Geometry: final body of the model. Coordinates: model frame, mm. Face numbers are marked on the shaded views. Round coordinates to 2 decimals unless told otherwise and drop trailing zeros. Loops run counter-clockwise (first coordinate to the right, second up) from the corner with the lowest first, then second, coordinate; pieces in that order, holes last. Notation, with made-up numbers: (-36.75, 62.5) -> (10.25, 62.5) arc R16 ccw to (10.25, 67.5) -> close; hole circle Ø9 at (48, -36.5). An arc over 180 degrees is marked (long way). Answer in a Markdown table with one row per item.
```python
from build123d import *

# Parameters (mm, degrees)
SKETCH2_R             = 7.9375
SKETCH2_R_2           = 3.8862
BOSS_EXTRUDE1_DEPTH   = 6.35
SKETCH2_R_3           = 1.70815
BOSS_EXTRUDE1_2_DEPTH = 6.35
BOSS_EXTRUDE3_START   = -2.54
SKETCH2_6_R           = 7.9375
SKETCH2_6_R_2         = 1.70815
BOSS_EXTRUDE3_DEPTH   = 2.54
CHAMFER2_SIZE         = 1.27
CHAMFER2_SIZE2        = 1.513527063
CHAMFER3_SIZE         = 0.635


with BuildPart() as part:
    # Sketch2 → Boss-Extrude1 (new body)
    with BuildSketch(Plane(origin=(0, 0, 0), x_dir=(0, 1, 0), z_dir=(0, 0, 1))):
        with Locations(Location((0, 0, 0), (0, 0, 270))):
            Circle(SKETCH2_R)
        with Locations(Location((0, 0, 0), (0, 0, 270))):
            Circle(SKETCH2_R_2, mode=Mode.SUBTRACT)
    extrude(amount=BOSS_EXTRUDE1_DEPTH)

    # Sketch2<6> → Boss-Extrude3 (add)
    with BuildSketch(Plane(origin=(0, 0, 0), x_dir=(0, 1, 0), z_dir=(0, 0, 1)).offset(BOSS_EXTRUDE3_START)):
        with Locations(Location((0, 0, 0), (0, 0, 270))):
            Circle(SKETCH2_6_R)
        with Locations(Location((0, 0, 0), (0, 0, 270))):
            Circle(SKETCH2_6_R_2, mode=Mode.SUBTRACT)
    extrude(amount=BOSS_EXTRUDE3_DEPTH)

    # Chamfer2
    chamfer2_edges = [part.edges().sort_by_distance(p)[0] for p in [
        (-1.70815, 0, -2.54),
    ]]
    chamfer2_side = [part.faces().sort_by_distance(p)[0] for p in [
        (-1.70815, 0, -1.27),
    ]]
    chamfer(chamfer2_edges, length=CHAMFER2_SIZE, length2=CHAMFER2_SIZE2, reference=chamfer2_side[0])

    # Chamfer3
    chamfer3_edges = [part.edges().sort_by_distance(p)[0] for p in [
        (-7.9375, 0, 6.35),
        (-7.9375, 0, -2.54),
        (-3.8862, 0, 6.35),
    ]]
    chamfer(chamfer3_edges, length=CHAMFER3_SIZE)


with BuildPart() as body_2:
    # Sketch2 → Boss-Extrude1 2 (new body)
    with BuildSketch(Plane(origin=(0, 0, 0), x_dir=(0, 1, 0), z_dir=(0, 0, 1))):
        with Locations(Location((0, 0, 0), (0, 0, 270))):
            Circle(SKETCH2_R_3)
    extrude(amount=BOSS_EXTRUDE1_2_DEPTH)


solid = part.part
```
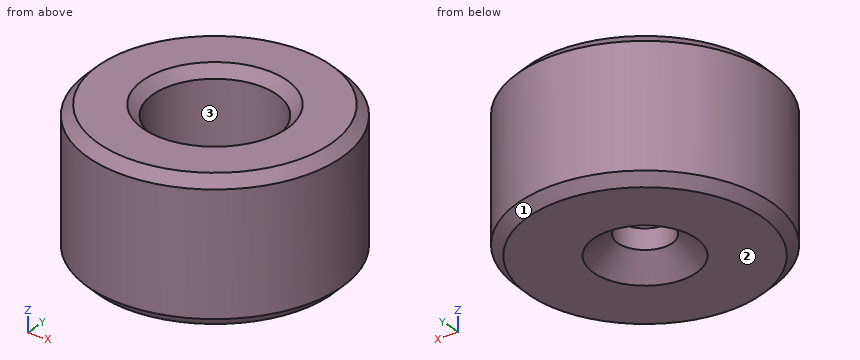
Item 1: Section query D-D, the plane z = -0.25. Output: boundary loops of the cut face in (x, y) (1 decimal), and give its area (3 significant figures).
Ans:
| item | result |
|---|---|
| outline | circle Ø15.9 at (0, 0); hole circle Ø3.4 at (0, 0) |
| area | 189 mm2 |
Item 2: Section query C-C, the plane z = 2. Output: boundary loops of the cut face in (x, y) (1 decimal).
Ans:
| item | result |
|---|---|
| outline | circle Ø15.9 at (0, 0); hole circle Ø7.8 at (0, 0) |
Item 3: Ray query, L1, parallel to Y at x = 0, z = -0.65; L2, parallel to Y at x = 0, z = 3; L3, parallel to X at y = 2.5, z = 5.5. Return the intervals inside material, ascending.
Ans:
| item | result |
|---|---|
| L1 | -7.94 to -1.71, 1.71 to 7.94 |
| L2 | -7.94 to -3.89, 3.89 to 7.94 |
| L3 | -7.53 to -2.98, 2.98 to 7.53 |
Item 4: First-contact query: P1, Ø1, axis at x = 2, z = 1, coming from the +Y side; P2, Ø1.5, axis at x = 2, y = 0, coming from the +Z side; P3, Ø5.5, axis at x = 0, y = 0, coming from the -Z side. Flat tips, straight axial feed; report the tip coordinate or a pass-through.
Ans:
| item | result |
|---|---|
| P1 | y = 7.79 |
| P2 | z = 0 |
| P3 | z = -2.14 |
Item 5: Mould query, pull axis X, two halves, no side actions, for the marked faces 1, 2 and 3. Classes: released by +X, released by -X, zero draft, split by the parting line, or undercut.
Ans:
| item | result |
|---|---|
| face 1 | split by the parting line |
| face 2 | zero draft |
| face 3 | undercut |
